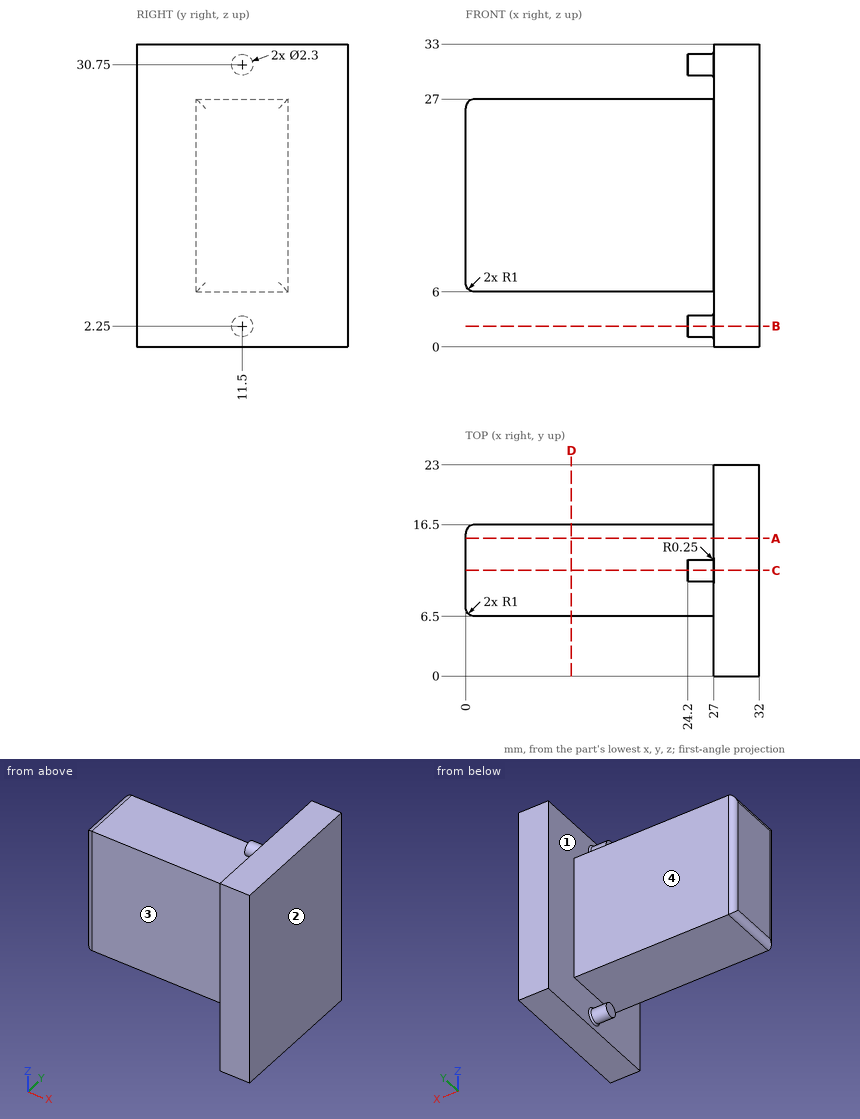
For this review, use the dimensioned drawing (mm, ordinates from the lowest corner) and the shaded views. A direction names the side the tool comes from. Round coordinates to 2 decimals unless told otherwise and drop trailing zeros. Write each loop counter-clockwise with the first axis right and the second up, starting at its lowest first coordinate (ties: lowest second). Pieces come first, ordered by that corner, then holes. Notation, with made-up numbers: M 47,-25 L 104,-25 A31 ccw 104,1 Z; hole C 19,-24 d9. An arc over 180 degrees is marked long. Write item = value, one per line. Start each with the question number.
(1) We need section D-D (x = 11.5). Give the boundary of the cut face in (y, z), then the cut area to 3 significant figures.
(2) Clearance check with flat-ended pins moving along their axes: pin 1 Ø12 at (x, y) = (10.5, 17) entering from +Z; pin 2 Ø10 at (x, y) = (16.5, 18) entering from -Z; pin 3 Ø5 at (x, z) = (19.5, 11.5) entering from +Y; pin 4 Ø17 at (x, z) = (19.5, 12) entering from +Y. State where each tip first meets the part, or that it passes through.
(3) We need section C-C (y = 11.5). Give the boundary of the cut face in (x, z), then the cut area to 3 significant figures.
(4) For line 1 along Y through (x, z) = (18, 10); line 2 along X through (y, z) = (17.5, 15); line 3 along Z through (x, y) = (16, 13), list the stretches that pass through material, from the lowest coordinate up.
(5) We need section B-B (z = 2.25). Give the boundary of the cut face in (x, y), then the cut area to 3 significant figures.
(6) For the marked faces 1, 2, 3 and 4, list the 3-axis set-ups (+Z, -Z, +X, -X, +Y, -Y) from which the entire face can be reached by the end or side of a thin tool; tool diameter is ignored.
(7) We need section A-A (y = 15). Give the boundary of the cut face in (x, z), then the cut area to 3 significant figures.
Results found:
q1.outline = M 6.5,6 L 16.5,6 L 16.5,27 L 6.5,27 Z
q1.area = 210 mm²
q2.pin_1 = 27
q2.pin_2 = 6
q2.pin_3 = 16.5
q2.pin_4 = 23
q3.outline = M 0,7 A1 ccw 1,6 L 27,6 L 27,3.65 A0.25 cw 26.75,3.4 L 24.2,3.4 L 24.2,1.1 L 26.75,1.1 A0.25 cw 27,0.85 L 27,0 L 32,0 L 32,33 L 27,33 L 27,32.15 A0.25 cw 26.75,31.9 L 24.2,31.9 L 24.2,29.6 L 26.75,29.6 A0.25 cw 27,29.35 L 27,27 L 1,27 A1 ccw 0,26 Z
q3.area = 745 mm²
q4.line_1 = 6.5 to 16.5
q4.line_2 = 27 to 32
q4.line_3 = 6 to 27
q5.outline = M 24.2,10.35 L 26.75,10.35 A0.25 cw 27,10.1 L 27,0 L 32,0 L 32,23 L 27,23 L 27,12.9 A0.25 cw 26.75,12.65 L 24.2,12.65 Z
q5.area = 121 mm²
q6.face_1 = -X
q6.face_2 = +Z, -Z, +X, +Y, -Y
q6.face_3 = +Z, -Z, -X, -Y
q6.face_4 = +Z, -Z, -X, +Y
q7.outline = M 0,7 A1 ccw 1,6 L 27,6 L 27,0 L 32,0 L 32,33 L 27,33 L 27,27 L 1,27 A1 ccw 0,26 Z
q7.area = 732 mm²
